Source: three-view drawing plus pictorial views. Frame: mm from the lowest corner of the part. A direction names the side the tool comes from. Coordinates: 2 decimals unless noted, no trailing zeros. Order: outer loops, then holes, each group sorted by start corner. A loop starts at its lowest first (then second) coordinate and runs counter-clockwise, first axis right, second up. Notation, with made-up numbers: (33, 33) - (85, 33) arc R24 cw to (85, 56) - close; hole circle Ø1 at (-20, 46.5). An arc over 180 degrees is marked (long way). Use a Markdown table: item, result. Add a question column.
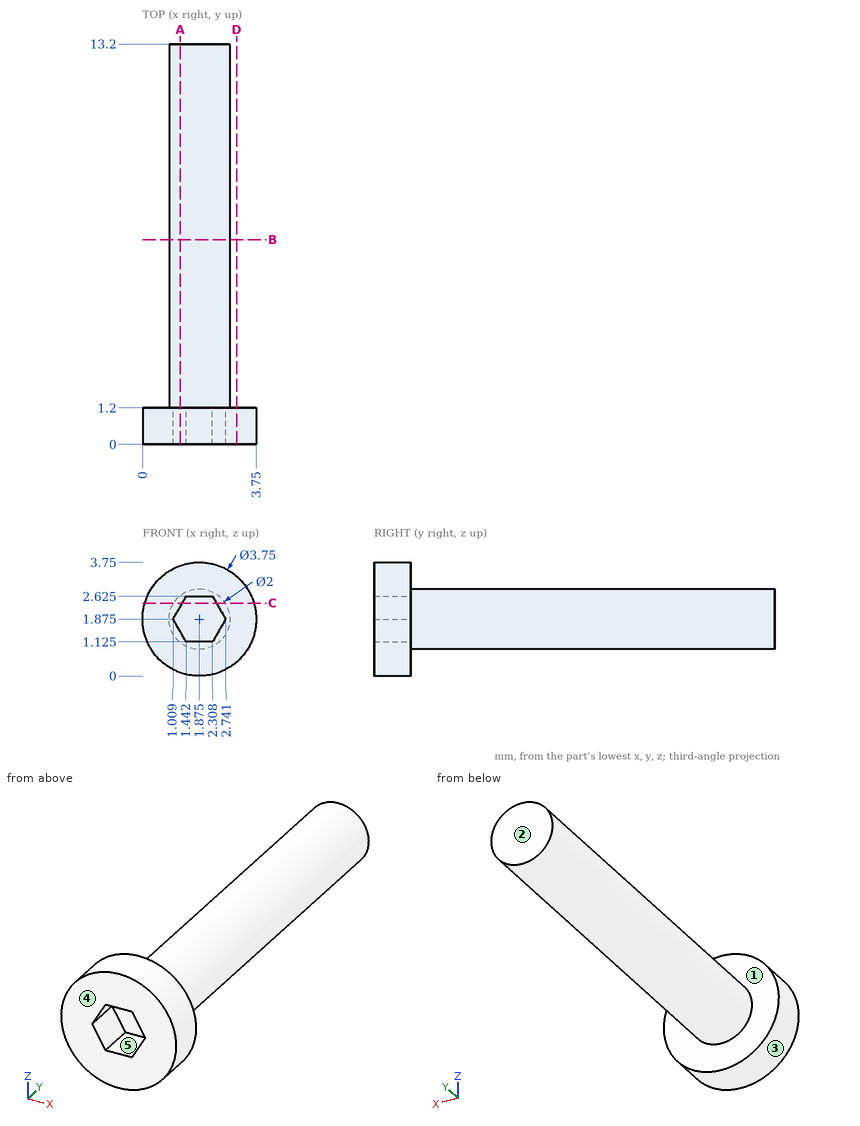
1) Section B-B (y = 6.75). Return loops of the section in (x, z) (3 decimals).
2) Ray query, line 1 along Y through (x, z) = (0.85, 3.25); line 2 along X through (y, z) = (5.75, 1.95); line 3 along Y through (x, z) = (1.8, 1.35). Return the intervals inside material, ascending.
3) Pin query (flat end, axial travel): pin 1 (2 mm diameter, centred on x = 2.5, y = 8.5, fed in from +Z) (3 decimals). Return the tip coordinate at first contact, or that it passes through.
4) Section D-D (x = 3.1). Return loops of the section in (y, z), then the cut area to 3 significant figures.
5) Section C-C (z = 2.4). Return loops of the section in (x, y) (3 decimals), then the cut area to 3 significant figures.
6) Set-up query: the marked faces 1 and 2. Return all of +Z, -Z, +X, -X, +Y, -Y with unobstructed straight access to the full face (end or side cutting, diameter ignored); none if empty.
7) Section A-A (x = 1.25). Return loops of the section in (y, z).
8) Draft query along Z for the marked faces 3, 4 and 5. Return one class per face: pulls with the +Z half, pulls with the -Z half, needs draft (parallel to the pull), parting line crosses it, or undercut.
Values follow:
| question | item | result |
|---|---|---|
| 1 | outline | circle Ø2 at (1.875, 1.875) |
| 2 | line 1 | y = 0 to 1.2 |
| 2 | line 2 | x = 0.88 to 2.87 |
| 2 | line 3 | y = 1.2 to 13.2 |
| 3 | pin 1 | stops at z = 2.875 |
| 4 | outline | (0, 0.46) - (1.2, 0.46) - (1.2, 3.29) - (0, 3.29) - close |
| 4 | area | 3.41 mm² |
| 5 | outline | (0.075, 0) - (1.312, 0) - (1.312, 1.2) - (2.438, 1.2) - (2.438, 0) - (3.675, 0) - (3.675, 1.2) - (2.726, 1.2) - (2.726, 13.2) - (1.024, 13.2) - (1.024, 1.2) - (0.075, 1.2) - close |
| 5 | area | 23.4 mm² |
| 6 | face 1 | +Y |
| 6 | face 2 | +Z, -Z, +X, -X, +Y |
| 7 | outline | (0, 0.11) - (1.2, 0.11) - (1.2, 1.09) - (13.2, 1.09) - (13.2, 2.66) - (1.2, 2.66) - (1.2, 3.64) - (0, 3.64) - (0, 2.29) - (1.2, 2.29) - (1.2, 1.46) - (0, 1.46) - close |
| 8 | face 3 | parting line crosses it |
| 8 | face 4 | needs draft |
| 8 | face 5 | undercut |
